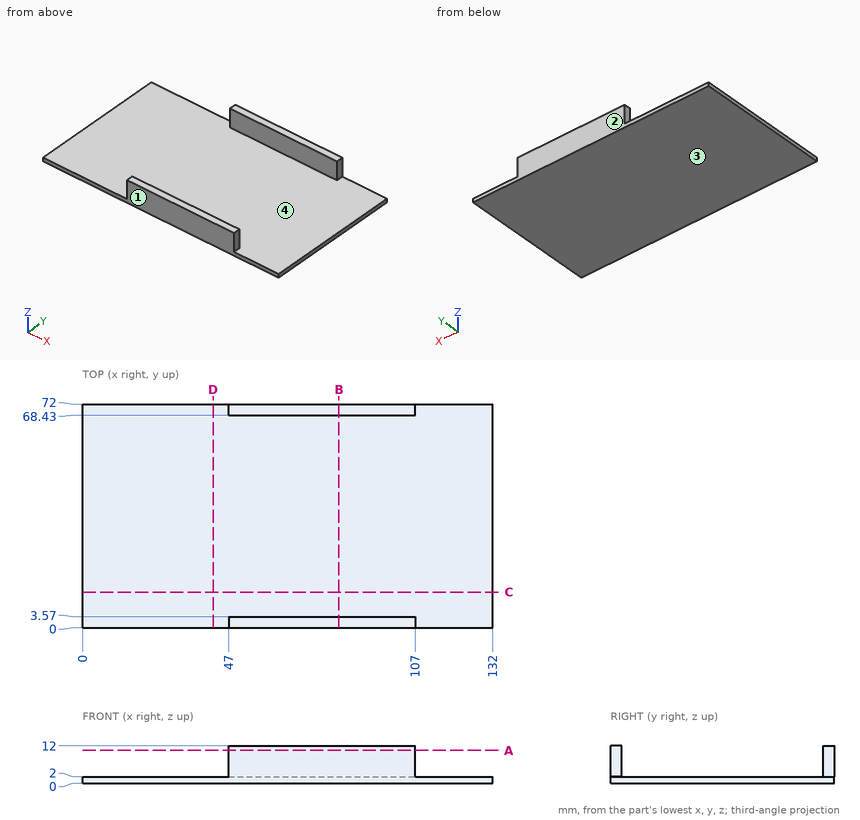
Geometry check sheet. Reference: drawing and pictorial views, mm from the part's lowest x, y, z. Give positions to 0.01 mm unless a question says otherwise; leave off trailing zeros. Write each loop counter-clockwise with the first axis right and the second up, starting at its lowest first coordinate (ties: lowest second). Pieces come first, ordered by that corner, then holes. Notation, with made-up numbers: (62.25, 37.25) -> (79.25, 37.25) arc R18 cw to (79.25, 70.25) -> close; hole circle Ø9 at (58.5, -1). An arc over 180 degrees is marked (long way). One line per item, written item: value. Start each with the question number.
Item 1: Gauge pin test, flat ends, axial feed: pin 1 (2 mm diameter, centred on x = 67, y = 36.5, fed in from +Z); pin 2 (4 mm diameter, centred on y = 70, z = 8.5, fed in from +X); pin 3 (1.1 mm diameter, centred on y = 70.5, z = 5, fed in from -X). Record the tip position at first contact, or that the pin passes through.
Item 2: Section check B-B on x = 82.5. Record the cut outline in (y, z).
Item 3: Section check D-D on x = 42. Record the cut outline in (y, z).
Item 4: Material ranges on probe 1 along Y at (x, z) = (84, 3.25); probe 2 along Z at (x, y) = (38.5, 35.5), recorded low to high. Write a range as from..to.
Item 5: Draft check along Y on the marked faces 1, 2, 3 and 4. Enter one of: +Y half, -Y half, draft (parallel to the pull), parting line (faces both ways), or undercut.
Item 6: Section check A-A on z = 10.5. Record the cut outline in (x, y).
Item 7: Section check C-C on y = 11.5. Record the cut outline in (x, z).
Results list:
1. pin 1: z = 2
1. pin 2: x = 107
1. pin 3: x = 47
2. outline: (0, 0) -> (72, 0) -> (72, 12) -> (68.43, 12) -> (68.43, 2) -> (3.57, 2) -> (3.57, 12) -> (0, 12) -> close
3. outline: (0, 0) -> (72, 0) -> (72, 2) -> (0, 2) -> close
4. probe 1: 0..3.57, 68.43..72
4. probe 2: 0..2
5. face 1: -Y half
5. face 2: +Y half
5. face 3: draft
5. face 4: undercut
6. outline: (47, 0) -> (107, 0) -> (107, 3.57) -> (47, 3.57) -> close; (47, 68.43) -> (107, 68.43) -> (107, 72) -> (47, 72) -> close
7. outline: (0, 0) -> (132, 0) -> (132, 2) -> (0, 2) -> close
